from build123d import *

# Parameters (mm, degrees)
F1_DEPTH = 25.4
F2_D     = 10.16


with BuildPart() as f1:
    # F0 (on Top) → F1 (new body)
    with BuildSketch(Plane.XY):
        with BuildLine():
            add(Edge.make_bspline(
                [(-13.7100163847, 12.9788173363), (-12.4863722513, 11.5414430545), (-10.1918765367, 8.8461748471), (-10.7057072132, 4.2242559095), (-13.3579996874, 1.4923212615), (-14.8068163544, 0)],
                knots=[0, 0, 0, 0, 0.3414517803, 0.6402675625, 1, 1, 1, 1], degree=3))
            ThreePointArc((-14.8068163544, 0), (0.3655990586, -33.5925494725), (15.5380144715, 0))
            add(Edge.make_bspline(
                [(13.7100145221, 13.3444173262), (11.9781094837, 11.9335853093), (8.8109129891, 9.353546497), (10.0241222697, 4.4047922136), (13.5389223726, 1.5969817671), (15.5380144715, 0)],
                knots=[0, 0, 0, 0, 0.3422584436, 0.6259002191, 1, 1, 1, 1], degree=3))
            ThreePointArc((13.7100145221, 13.3444173262), (-0.3197104944, 37.1398622542), (-13.7100163847, 12.9788173363))
        make_face()
    extrude(amount=F1_DEPTH)

    # F2 (through all)
    with Locations(Plane(origin=(0, 0, 0), x_dir=(1, 0, 0), z_dir=(0, 0, -1))):
        with Locations((-0.1075960341, -21.2312593567)):
            Hole(F2_D / 2)


solid = f1.part
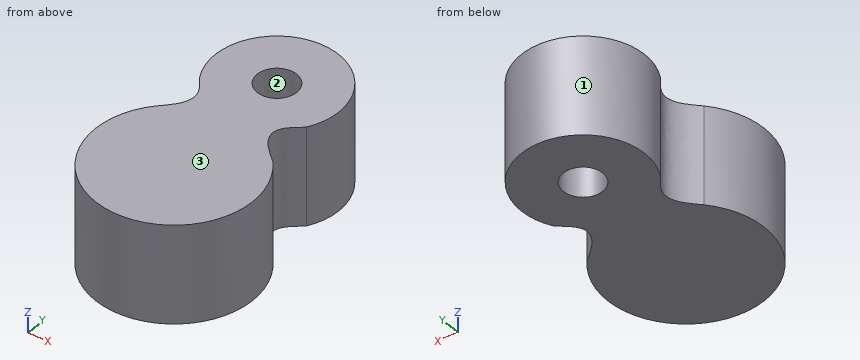
Source: CAD feature listing. Evaluate the final solid. Frame: model axes, mm. Face numbers are marked on the shaded views. Give positions to 0.01 mm unless a question says otherwise; leave off trailing zeros. Loops run counter-clockwise (first coordinate to the right, second up) from the corner with the lowest first, then second, coordinate; pieces in that order, holes last. Notation, with made-up numbers: (75, 67.5) -> (93, 67.5) arc R13 ccw to (93, 82.5) -> close; hole circle Ø6 at (-11.75, 17). An arc over 180 degrees is marked (long way). Use a Markdown table: item, result. Add a question column.
1) Section query A-A, the plane y = 17.5. Return the cut outline in (x, z).
2) Line query: line 1 along X through (y, z) = (21.5, 6.75); line 2 along Y through (x, z) = (-12.5, 24.75); line 3 along Y through (x, z) = (1.5, 14.5). Output: solid intervals per line, ascending. Write a range as [from, to].
3) Section query B-B, the plane y = 25. Return the cut outline in (x, z).
4) Section query C-C, the plane x = -9. Return the cut outline in (y, z), then the cut area to 3 significant figures.
5) First-contact query: pin 1 (6 mm diameter, centred on x = 1, y = 0.5, fed in from -Z); pin 2 (8 mm diameter, centred on y = 3.5, z = 13, fed in from -X); pin 3 (1 mm diameter, centred on y = -18.5, z = 12, fed in from +X); pin 4 (2 mm diameter, centred on x = 13, z = 4, fed in from -Y). Flat tips, straight axial feed; report the tip coordinate or a pass-through.
6) Section query D-D, the plane y = -9.5. Return the cut outline in (x, z).
7) Pull-direction query (Y, two-part tool) for the marked faces 1, 2 and 3; classes: +Y half, -Y half, draft (parallel to the pull), parting line (faces both ways), or undercut.
Numbers:
| question | item | result |
|---|---|---|
| 1 | outline | (-15.57, 0) -> (-3.55, 0) -> (-3.55, 25.4) -> (-15.57, 25.4) -> close; (3.34, 0) -> (15.36, 0) -> (15.36, 25.4) -> (3.34, 25.4) -> close |
| 2 | line 1 | x = [-16.02, -5.18], [4.97, 15.8] |
| 2 | line 2 | y = [-28.97, 2.52], [11.52, 31.21] |
| 2 | line 3 | y = [-33.56, 16.41], [26.05, 37.06] |
| 3 | outline | (-15.56, 0) -> (-3.51, 0) -> (-3.51, 25.4) -> (-15.56, 25.4) -> close; (3.3, 0) -> (15.35, 0) -> (15.35, 25.4) -> (3.3, 25.4) -> close |
| 4 | outline | (-31.29, 0) -> (34.42, 0) -> (34.42, 25.4) -> (-31.29, 25.4) -> close |
| 4 | area | 1,670 mm2 |
| 5 | pin 1 | stops at z = 0 |
| 5 | pin 2 | stops at x = -15.23 |
| 5 | pin 3 | stops at x = 20.05 |
| 5 | pin 4 | stops at y = -29.91 |
| 6 | outline | (-19.48, 0) -> (20.21, 0) -> (20.21, 25.4) -> (-19.48, 25.4) -> close |
| 7 | face 1 | undercut |
| 7 | face 2 | undercut |
| 7 | face 3 | draft |
